from build123d import *

# Parameters (mm, degrees)
F0_R          = 6
F1_DEPTH      = 35
F1_DEPTH_BACK = 12
F2_W          = 45
F2_H          = 20
F3_DEPTH      = 80


with BuildPart() as f1:
    # F0 (on Top) → F1 (new body, two sides)
    with BuildSketch(Plane.XY) as f1_sk:
        Polygon((30, 30), (30, 52.5), (-30, 52.5), (-30, 30), (-52.5, 30), (-52.5, -30), (-30, -30), (-30, -52.5), (30, -52.5), (30, -30), (52.5, -30), (52.5, 30), align=None)
        with Locations((-36, -15)):
            Circle(F0_R, mode=Mode.SUBTRACT)
        with Locations((36, -15)):
            Circle(F0_R, mode=Mode.SUBTRACT)
        with Locations((-36, 15)):
            Circle(F0_R, mode=Mode.SUBTRACT)
        with Locations((36, 15)):
            Circle(F0_R, mode=Mode.SUBTRACT)
    extrude(amount=F1_DEPTH)
    extrude(f1_sk.sketch, amount=-F1_DEPTH_BACK)

    # F2 (on face) → F3 (cut)
    with BuildSketch(Plane.XZ.offset(52.5)):
        with Locations((-0.129311, 25)):
            Rectangle(F2_W, F2_H)
    extrude(amount=-F3_DEPTH, mode=Mode.SUBTRACT)


solid = f1.part
Read the model definition and answer for the solid it produces. Units are mm, in the model's axes. A direction names the side the tool comes from. Give positions to 0.01 mm unless a question says otherwise; leave off trailing zeros. Write each loop counter-clockwise with the first axis right and the second up, starting at its lowest first coordinate (ties: lowest second). Pieces come first, ordered by that corner, then holes. Notation, with made-up numbers: (-2, -7) - (25, -7) arc R18 cw to (25, 25) - close; hole circle Ø2 at (51.25, 40.5). An arc over 180 degrees is marked (long way). Use CSV: the item, a comma, the result in double quotes. Start each with the question number.
Item 1: The mould has two halves that part along X. Classify faces 6 (the flat face through (-30, 41, 12)), 7 (the flat face through (52.5, 0, 12)), 8 (the flat face through (-22.629, -13, 25)), 9 (the flat face through (0, -52.5, 7)): pulls with the +X half, pulls with the -X half, needs draft (parallel to the pull), parting line crosses it, or undercut.
Item 2: Consider line 1 (Y direction, x = 36, z = -6); line 2 (X direction, y = -25.5, z = 29); line 3 (X direction, y = -17.5, z = 7.5). Determine where each line is inside the solid, lowest interval first.
Item 3: The part is cut by section D-D, the plane y = -26.5. Give the vertices of the cut face in (x, z), and give its area (4 significant figures).
Item 4: The part is cut by section A-A, the plane y = -15. Give the vertices of the cut face in (x, z), and give its area (3 significant figures).
Item 5: The part is cut by section B-B, the plane x = -36. Give the vertices of the cut face in (y, z), and give its area (3 significant figures).
Item 6: For faces 1 (the flat face through (0, 27.5, 25)), 2 (the flat face through (30, 41, 12)), 3 (the flat face through (-41, -30, 12)), 4 (the flat face through (-41, 30, 12)), 5 (the flat face through (41, -30, 12)), determine the directions among +Z, -Z, +X, -X, +Y, -Y from which every point of the face is accessible in a straight line to the end or side of a thin tool.
Item 7: The part is cut by section C-C, the plane z = 13.5. Give the vertices of the cut face in (x, y), and give its area (3 significant figures).
Item 8: Flat-ended cylindrical pins translate along their axes: P1, Ø7, axis at x = 36, y = -15, coming from the -Z side; P2, Ø7, axis at y = 41, z = 12, coming from the +X side; P3, Ø10, axis at x = 10, z = 24.5, coming from the -Y side; P4, Ø19, axis at x = -36, y = 15, coming from the -Z side. Find the tip coordinate at first contact, or state that the pin passes through.
Taken from the geometry:
1,face 6,"pulls with the -X half"
1,face 7,"pulls with the +X half"
1,face 8,"undercut"
1,face 9,"needs draft"
2,line 1,"-30 to -21, -9 to 9, 21 to 30"
2,line 2,"-52.5 to -22.63, 22.37 to 52.5"
2,line 3,"-52.5 to -41.45, -30.55 to 30.55, 41.45 to 52.5"
3,outline,"(-52.5, -12) - (52.5, -12) - (52.5, 35) - (22.37, 35) - (22.37, 15) - (-22.63, 15) - (-22.63, 35) - (-52.5, 35) - close"
3,area,"4,035 mm2"
4,outline,"(-52.5, -12) - (-42, -12) - (-42, 35) - (-52.5, 35) - close; (-30, -12) - (30, -12) - (30, 35) - (22.37, 35) - (22.37, 15) - (-22.63, 15) - (-22.63, 35) - (-30, 35) - close; (42, -12) - (52.5, -12) - (52.5, 35) - (42, 35) - close"
4,area,"2,910 mm2"
5,outline,"(-30, -12) - (-21, -12) - (-21, 35) - (-30, 35) - close; (-9, -12) - (9, -12) - (9, 35) - (-9, 35) - close; (21, -12) - (30, -12) - (30, 35) - (21, 35) - close"
5,area,"1,690 mm2"
6,face 1,"+Z, -Y"
6,face 2,"+Z, -Z, +X, +Y"
6,face 3,"+Z, -Z, -X, -Y"
6,face 4,"+Z, -Z, -X, +Y"
6,face 5,"+Z, -Z, +X, -Y"
7,outline,"(-52.5, -30) - (-30, -30) - (-30, -52.5) - (30, -52.5) - (30, -30) - (52.5, -30) - (52.5, 30) - (30, 30) - (30, 52.5) - (-30, 52.5) - (-30, 30) - (-52.5, 30) - close; hole circle Ø12 at (-36, -15); hole circle Ø12 at (-36, 15); hole circle Ø12 at (36, -15); hole circle Ø12 at (36, 15)"
7,area,"8,550 mm2"
8,P1,"through"
8,P2,"x = 30"
8,P3,"y = 27.5"
8,P4,"z = -12"
